```python
from build123d import *

# Parameters (mm, degrees)
EXTRUDE_1_DEPTH          = 57
CUT_EXTRUDE_1_DEPTH      = 57
CUT_EXTRUDE_2_DEPTH      = 57
SKETCH_5_R               = 7.5
SKETCH_5_R_2             = 1.25
CUT_EXTRUDE_3_DEPTH      = 57
PATTERN_CIRCULAR_1_COUNT = 6
SKETCH_6_R               = 12.5
SKETCH_6_R_2             = 1.25
CUT_EXTRUDE_4_DEPTH      = 57
PATTERN_CIRCULAR_2_COUNT = 4
SKETCH_7_R               = 1.25
CUT_EXTRUDE_5_DEPTH      = 10
PATTERN_CIRCULAR_3_COUNT = 3
PATTERN_CIRCULAR_3_ANGLE = 180


with BuildPart() as part:
    # 草图1 → 凸台-拉伸1 (new body)
    with BuildSketch(Plane.XY):
        Polygon((0, 67), (0, 0), (57, 0), (57, 4), (4, 4), (4, 67), align=None)
    extrude(amount=EXTRUDE_1_DEPTH)

    # 草图3 → 切除-拉伸1 (cut)
    with BuildSketch(Plane.XZ):
        with BuildLine():
            Line((57, 57), (28.5, 57))
            ThreePointArc((28.5, 57), (48.652543264, 48.652543264), (57, 28.5))
            Line((57, 28.5), (57, 57))
        make_face()
        with BuildLine():
            ThreePointArc((57, 28.5), (48.652543264, 8.347456736), (28.5, 0))
            Line((28.5, 0), (57, 0))
            Line((57, 0), (57, 28.5))
        make_face()
    extrude(amount=-CUT_EXTRUDE_1_DEPTH, mode=Mode.SUBTRACT)

    # 草图4 → 切除-拉伸2 (cut)
    with BuildSketch(Plane.ZY):
        with BuildLine():
            Line((57, 67), (28.5, 67))
            ThreePointArc((28.5, 67), (48.652543264, 58.652543264), (57, 38.5))
            Line((57, 38.5), (57, 67))
        make_face()
        with BuildLine():
            Line((28.5, 67), (0, 67))
            Line((0, 67), (0, 38.5))
            ThreePointArc((0, 38.5), (8.347456736, 58.652543264), (28.5, 67))
        make_face()
    extrude(amount=-CUT_EXTRUDE_2_DEPTH, mode=Mode.SUBTRACT)

    # 草图5 → 切除-拉伸3 (cut)
    with BuildSketch(Plane.ZY):
        with Locations((28.5, 38.5)):
            Circle(SKETCH_5_R)
        with Locations((42, 38.5)):
            Circle(SKETCH_5_R_2)
    cut_extrude_3 = extrude(amount=-CUT_EXTRUDE_3_DEPTH, mode=Mode.SUBTRACT)

    # 阵列(圆周)1: 切除-拉伸3 ×6 about axis
    pattern_circular_1_axis = Axis((0, 38.5, 28.5), (1, 0, 0))
    for i in range(1, PATTERN_CIRCULAR_1_COUNT):
        add(cut_extrude_3.rotate(pattern_circular_1_axis, i * 360 / PATTERN_CIRCULAR_1_COUNT), mode=Mode.SUBTRACT)

    # 草图6 → 切除-拉伸4 (cut)
    with BuildSketch(Plane.XZ):
        with Locations(Location((28.5, 28.5, 0), (0, 0, 270))):
            Circle(SKETCH_6_R)
        with Locations(Location((41.935028843, 41.935028843, 0), (0, 0, 270))):
            Circle(SKETCH_6_R_2)
    cut_extrude_4 = extrude(amount=-CUT_EXTRUDE_4_DEPTH, mode=Mode.SUBTRACT)

    # 阵列(圆周)2: 切除-拉伸4 ×4 about axis
    pattern_circular_2_axis = Axis((28.5, 0, 28.5), (0, 1, 0))
    for i in range(1, PATTERN_CIRCULAR_2_COUNT):
        add(cut_extrude_4.rotate(pattern_circular_2_axis, i * 360 / PATTERN_CIRCULAR_2_COUNT), mode=Mode.SUBTRACT)

    # 草图7 → 切除-拉伸5 (cut)
    with BuildSketch(Plane.ZY):
        with Locations((51, 38.5)):
            Circle(SKETCH_7_R)
    cut_extrude_5 = extrude(amount=-CUT_EXTRUDE_5_DEPTH, mode=Mode.SUBTRACT)

    # 阵列(圆周)3: 切除-拉伸5 ×3 about axis
    pattern_circular_3_axis = Axis((0, 38.5, 28.5), (-1, 0, 0))
    for i in range(1, PATTERN_CIRCULAR_3_COUNT):
        add(cut_extrude_5.rotate(pattern_circular_3_axis, i * PATTERN_CIRCULAR_3_ANGLE / (PATTERN_CIRCULAR_3_COUNT - 1)), mode=Mode.SUBTRACT)


solid = part.part
```
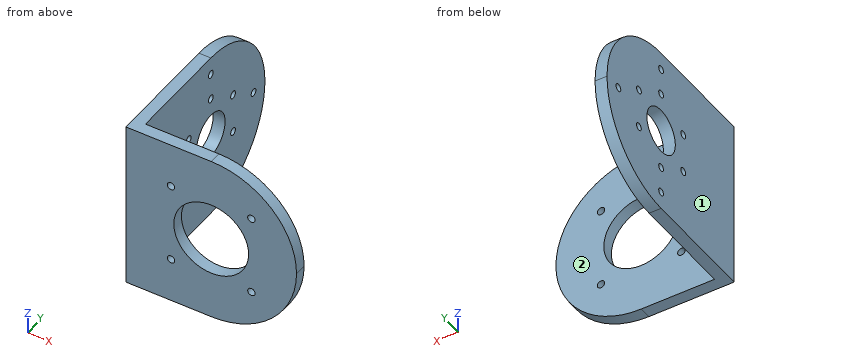
Here's how the part is built. I have some questions about the finished solid (model axes, mm). Face numbers are marked on the shaded views. A direction names the side the tool comes from. Coordinates: 2 decimals unless noted, no trailing zeros. Loops run counter-clockwise (first coordinate to the right, second up) from the corner with the lowest first, then second, coordinate; pieces in that order, holes last. Notation, with made-up numbers: (54.25, 62) - (108.25, 62) arc R31 ccw to (108.25, 90) - close; hole circle Ø5 at (22, 36.25). An arc over 180 degrees is marked (long way). Return JSON: item names as keys, results as strings. Group by question number.
Item 1: If we section it at B-B on z = 31.5: Write out the boundary of the cut face in (x, y), and give its area (3 significant figures).
Item 2: If we section it at C-C on x = 34: Write out the boundary of the cut face in (y, z), and give its area (3 significant figures).
Item 3: On a 3-axis mill with a long thin cutter (end or side, diameter ignored), from which of +Z, -Z, +X, -X, +Y, -Y can I reach the whole of each face in a straight line? I mean the marked faces 1 and 2. Say none if no direction works.
Item 4: If we section it at A-A on y = 61: Write out the boundary of the cut face in (x, z), and give its area (3 significant figures).
Item 5: I need wall thicknesses on line 1 (Y direction, x = 37, z = 40); line 2 (Y direction, x = 3, z = 35). Which ranges of each line are inside material? Lowest first, please. Write a range as from..to.
Item 6: If we section it at D-D on z = 38: Write out the boundary of the cut face in (x, y).
Item 7: Will these pins go through, and if not, where does the flat tip stop? P1, Ø3, axis at y = 38.5, z = 51, coming from the +X side; P2, Ø4, axis at x = 15.06, z = 15.06, coming from the +Y side.
Calculated:
{
 "1": {"outline": "(0, 0) - (16.37, 0) - (16.37, 4) - (4, 4) - (4, 31.63) - (0, 31.63) - close; (0, 45.37) - (4, 45.37) - (4, 66.84) - (0, 66.84) - close; (40.63, 0) - (56.84, 0) - (56.84, 4) - (40.63, 4) - close", "area": "327 mm^2"},
 "2": {"outline": "(0, 0.54) - (4, 0.54) - (4, 17.28) - (0, 17.28) - close; (0, 39.72) - (4, 39.72) - (4, 56.46) - (0, 56.46) - close", "area": "134 mm^2"},
 "3": {"face 1": "+Z, -Z, -X, +Y, -Y", "face 2": "+Z, -Z, +X, +Y"},
 "4": {"outline": "(0, 11.01) - (4, 11.01) - (4, 27.25) - (0, 27.25) - close; (0, 29.75) - (4, 29.75) - (4, 45.99) - (0, 45.99) - close", "area": "130 mm^2"},
 "5": {"line 1": "y = 0..4", "line 2": "y = 0..25.58, 28.03..34.76, 42.24..48.97, 51.42..66.25"},
 "6": {"outline": "(0, 0) - (20.38, 0) - (20.38, 4) - (4, 4) - (4, 65.37) - (0, 65.37) - close; (36.62, 0) - (55.37, 0) - (55.37, 4) - (36.62, 4) - close"},
 "7": {"P1": "stops at x = 4", "P2": "stops at y = 4"}
}
